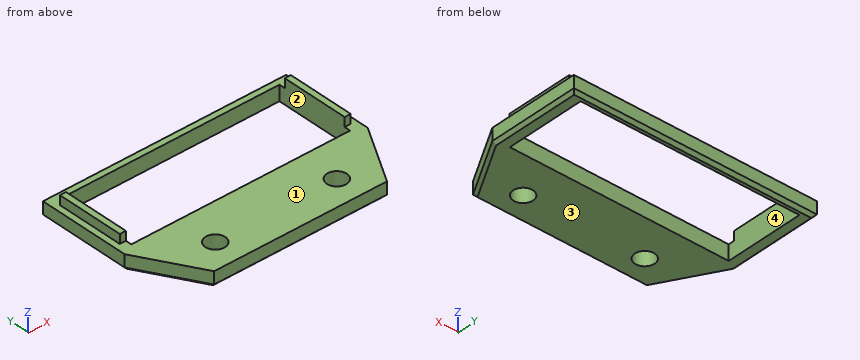
from build123d import *

# Parameters (mm, degrees)
F0_W     = 80
F0_H     = 30
F0_W_2   = 72
F0_H_2   = 26
F1_DEPTH = 5
F2_W     = 2
F2_H     = 22
F3_DEPTH = 3
F5_DEPTH = 5
F6_SIZE  = 1
F8_D     = 6.5
F9_D     = 6.5


with BuildPart() as f1:
    # F0 (on Top) → F1 (new body)
    with BuildSketch(Plane.XY):
        Rectangle(F0_W, F0_H)
        Rectangle(F0_W_2, F0_H_2, mode=Mode.SUBTRACT)
    extrude(amount=F1_DEPTH)

    # F2 (on face) → F3 (join)
    with BuildSketch(Plane.XY.offset(5)):
        with Locations((-37, 0)):
            Rectangle(F2_W, F2_H)
        with Locations((37, 0)):
            Rectangle(F2_W, F2_H)
    extrude(amount=F3_DEPTH)

    # F4 (on face) → F5 (join)
    with BuildSketch(Plane.XY.offset(5)):
        Polygon((40, -15), (-40, -15), (-28.4529946162, -35), (28.4529946162, -35), align=None)
    extrude(amount=-F5_DEPTH)

    # F6
    f6_edges = [f1.edges().sort_by_distance(p)[0] for p in [
        (0, 15, 0),
        (-40, 0, 0),
        (40, 0, 0),
        (34.226497, -25, 0),
        (0, -35, 0),
        (-34.226497, -25, 0),
    ]]
    chamfer(f6_edges, length=F6_SIZE)

    # F8 (through all)
    with Locations(Plane(origin=(0, 0, 0), x_dir=(1, 0, 0), z_dir=(0, 0, -1))):
        with Locations((20, 26)):
            Hole(F8_D / 2)

    # F9 (through all)
    with Locations(Plane(origin=(0, 0, 0), x_dir=(1, 0, 0), z_dir=(0, 0, -1))):
        with Locations((-20, 26)):
            Hole(F9_D / 2)


solid = f1.part
Here's how the part is built. I have some questions about the finished solid (model axes, mm). Face numbers are marked on the shaded views. A direction names the side the tool comes from. Coordinates: 2 decimals unless noted, no trailing zeros. Loops run counter-clockwise (first coordinate to the right, second up) from the corner with the lowest first, then second, coordinate; pieces in that order, holes last.
1. Imagine slicing it at C-C, the plane z = 3.5. Please give me the cut outline in (x, y), and give its area (3 significant figures).
2. If we mould it in two halves opening along X, with no side actions, what happens to the marked faces 1 and 2? For each: pulls with the +X half, pulls with the -X half, needs draft (parallel to the pull), parting line crosses it, or undercut.
3. For the marked faces 3 and 4, which set-ups out of +Z, -Z, +X, -X, +Y, -Y let a thin tool reach every point of the face, with its end or its side?
4. For P1, Ø0.6, axis at x = -37, z = 6, coming from the -Y side; P2, Ø10, axis at x = -27, y = -16, coming from the +Z side; P3, Ø0.6, axis at x = -36.5, z = 7, coming from the +Y side, each with a flat end and sliding along its axis, tell me the tip position at first contact or that it passes through.
5. I need wall thicknesses on L1, parallel to Y at x = 20, z = 2.9; L2, parallel to X at y = -26, z = 3.2; L3, parallel to Y at x = 23.5, z = 3.25. Which ranges of each line are inside material? Lowest first, please.
6. Imagine slicing it at A-A, the plane x = -20. Please give me the cut outline in (y, z), and give its area (3 significant figures).
7. Imagine slicing it at B-B, the plane y = 4.5. Please give me the cut outline in (x, z), and give its area (3 significant figures).
8. Imagine slicing it at D-D, the plane y = -26. Please give me the cut outline in (x, z).
Taken from the geometry:
1. outline: (-40, -15) - (-28.45, -35) - (28.45, -35) - (40, -15) - (40, 15) - (-40, 15) - close; hole (-36, -13) - (36, -13) - (36, 13) - (-36, 13) - close; hole circle Ø6.5 at (-20, -26); hole circle Ø6.5 at (20, -26)
1. area: 1,830 mm2
2. face 1: needs draft
2. face 2: undercut
3. face 3: -Z, +X, -X, +Y, -Y
3. face 4: +Z, -Z
4. P1: stops at y = -11
4. P2: stops at z = 5
4. P3: stops at y = 11
5. L1: y = -35 to -29.25, -22.75 to -13, 13 to 15
5. L2: x = -33.65 to -23.25, -16.75 to 16.75, 23.25 to 33.65
5. L3: y = -35 to -13, 13 to 15
6. outline: (-35, 1) - (-34, 0) - (-29.25, 0) - (-29.25, 5) - (-35, 5) - close; (-22.75, 0) - (-13, 0) - (-13, 5) - (-22.75, 5) - close; (13, 0) - (14, 0) - (15, 1) - (15, 5) - (13, 5) - close
6. area: 86.5 mm2
7. outline: (-40, 1) - (-39, 0) - (-36, 0) - (-36, 8) - (-38, 8) - (-38, 5) - (-40, 5) - close; (36, 0) - (39, 0) - (40, 1) - (40, 5) - (38, 5) - (38, 8) - (36, 8) - close
7. area: 51.0 mm2
8. outline: (-33.65, 1) - (-32.49, 0) - (-23.25, 0) - (-23.25, 5) - (-33.65, 5) - close; (-16.75, 0) - (16.75, 0) - (16.75, 5) - (-16.75, 5) - close; (23.25, 0) - (32.49, 0) - (33.65, 1) - (33.65, 5) - (23.25, 5) - close
